For this review, take the finished solid that the model builds, in its own axes (mm). Round coordinates to 2 decimals unless told otherwise and drop trailing zeros. Order: outer loops, then holes, each group sorted by start corner. A loop starts at its lowest first (then second) coordinate and runs counter-clockwise, first axis right, second up. Notation, with made-up numbers: (48.25, 27.25) -> (70.25, 27.25) arc R28 cw to (70.25, 45.25) -> close; hole circle Ø11 at (-21.75, 61.25). An arc over 180 degrees is marked (long way). Put each result on its own line as item: value. Start each with the question number.
```python
from build123d import *

# Parameters (mm, degrees)
FILLET1_R = 1
FILLET2_R = 50


with BuildPart() as part:
    # Sketch1 → Revolve1 (revolve)
    with BuildSketch(Plane.XY, mode=Mode.PRIVATE) as revolve1_sk:
        Polygon((0.875, 0.713567683), (4.425, 18), (4.425, 160.5), (0, 160.5), (0, 0.713567683), align=None)
    revolve(revolve1_sk.sketch.rotate(Axis((0, 160.5, 0), (0, -1, 0)), 90), axis=Axis((0, 160.5, 0), (0, -1, 0)))

    # Fillet1
    fillet1_edges = [part.edges().sort_by_distance(p)[0] for p in [
        (0, 0.713567683, -0.875),
    ]]
    fillet(fillet1_edges, radius=FILLET1_R)

    # Fillet2
    fillet2_edges = [part.edges().sort_by_distance(p)[0] for p in [
        (0, 18, -4.425),
    ]]
    fillet(fillet2_edges, radius=FILLET2_R)


solid = part.part
```
Item 1: For L1, parallel to Z at x = -0.5, y = 97.5; L2, parallel to X at y = 34.5, z = -0.25; L3, parallel to Z at x = 3.5, y = 114, list the stretches that pass through material, from the lowest coordinate up.
Item 2: Insertion check: pin 1 Ø4 at (x, y) = (2.5, 110.5) entering from +Z; pin 2 Ø4 at (y, z) = (36.5, -2.5) entering from +X; pin 3 Ø1 at (y, z) = (134, -3) entering from +X. Each pin has a flat end and moves straight along its axis. Give the tip position at first contact, or say it passes through.
Item 3: Consider section A-A, the plane y = 49. Write out the cut boundary in (x, z) (3 decimals).
Evaluation:
1. L1: z = -4.4 to 4.4
1. L2: x = -4.42 to 4.42
1. L3: z = -2.71 to 2.71
2. pin 1: stops at z = 4.4
2. pin 2: stops at x = 4.4
2. pin 3: stops at x = 3.65
3. outline: circle Ø8.85 at (0, 0)
